Could you check a few things on this model? Use its own coordinates, in mm. Face numbers are marked on the shaded views. A direction names the side the tool comes from. Coordinates: 2 decimals unless noted, no trailing zeros. Order: outer loops, then holes, each group sorted by start corner. A loop starts at its lowest first (then second) coordinate and runs counter-clockwise, first axis right, second up. Notation, with made-up numbers: (63, 9.5) - (112, 9.5) arc R23 ccw to (112, 34.5) - close; hole circle Ø4 at (6.25, -10). An arc over 180 degrees is marked (long way). One line per item, written item: value.
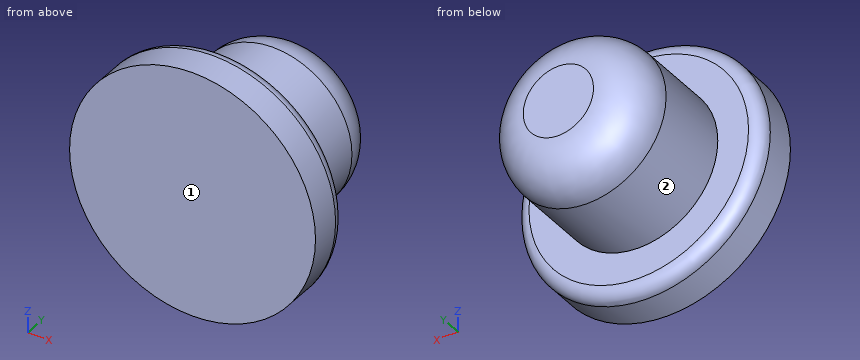
from build123d import *

# Parameters (mm, degrees)
SKETCH_1_R      = 2.8
EXTRUDE_2_DEPTH = 1
SKETCH_2_R      = 1.8
EXTRUDE_3_DEPTH = 2.8
FILLET_1_R      = 1
FILLET_2_R      = 0.3


with BuildPart() as part:
    # 草图1 → 凸台-拉伸2 (new body)
    with BuildSketch(Plane(origin=(0, 0, 0), x_dir=(1, 0, 0), z_dir=(0, 1, 0))):
        with Locations(Location((0, 0, 0), (0, 0, 270))):
            Circle(SKETCH_1_R)
    extrude(amount=EXTRUDE_2_DEPTH)

    # 草图2 → 凸台-拉伸3 (add)
    with BuildSketch(Plane(origin=(0, 1, 0), x_dir=(1, 0, 0), z_dir=(0, 1, 0))):
        with Locations(Location((0, 0, 0), (0, 0, 270))):
            Circle(SKETCH_2_R)
    extrude(amount=EXTRUDE_3_DEPTH)

    # 圆角1
    fillet_1_edges = [part.edges().sort_by_distance(p)[0] for p in [
        (0, 3.8, -1.8),
    ]]
    fillet(fillet_1_edges, radius=FILLET_1_R)

    # 圆角2
    fillet_2_edges = [part.edges().sort_by_distance(p)[0] for p in [
        (0, 1, -2.8),
    ]]
    fillet(fillet_2_edges, radius=FILLET_2_R)


solid = part.part
Item 1: If I drill on probe 1 along Y at (x, z) = (1.2, 1.7); probe 2 along Y at (x, z) = (1.7, 0.1); probe 3 along Z at (x, y) = (-0.45, 0.25), over which ranges is the centre line in solid material (lowest first)?
Conclusion:
probe 1: 0 to 1
probe 2: 0 to 3.23
probe 3: -2.76 to 2.76
Item 2: I'm going to push a flat-ended pin straight in: pin 1 Ø2 at (x, y) = (0.5, 2.5) entering from +Z. Where does the tip first touch, or does it pass through?
Conclusion:
pin 1: z = 1.8
Item 3: I want a section at A-A on y = 2.25. Please give me the cut outline in (x, z).
Conclusion:
outline: circle Ø3.6 at (0, 0)
Item 4: For the marked faces 1 and 2, which set-ups out of +Z, -Z, +X, -X, +Y, -Y let a thin tool reach every point of the face, with its end or its side?
Conclusion:
face 1: +Z, -Z, +X, -X, -Y
face 2: +Y
